Check sheet for the modelled part. Datum: model origin and axes. Units: mm. A direction names the side the tool comes from. Give positions to 0.01 mm unless a question says otherwise; leave off trailing zeros. Loops run counter-clockwise (first coordinate to the right, second up) from the corner with the lowest first, then second, coordinate; pieces in that order, holes last. Notation, with made-up numbers: M -3.5,78.25 L 41.5,78.25 A14 ccw 41.5,89.25 Z; hole C 35.5,-1.5 d8. An arc over 180 degrees is marked long. Use one line per item in the form item = value.
Autodesk Inventor part; units mm, degrees
ref_plane "YZ Plane" through (0, 0, 0) normal (1, 0, 0) x (0, 1, 0)
ref_plane "XZ Plane" through (0, 0, 0) normal (0, 1, 0) x (-1, 0, 0)
ref_plane "XY Plane" through (0, 0, 0) normal (0, 0, 1) x (1, 0, 0)
sketch "スケッチ1" plane through (0, 0, 0) normal (0, 0, 1) x (1, 0, 0)
  line L0 (-16.25, -16.25) -> (16.25, -16.25) construction
  line L1 (16.25, -16.25) -> (16.25, 16.25) construction
  line L2 (16.25, 16.25) -> (-16.25, 16.25) construction
  line L3 (-16.25, 16.25) -> (-16.25, -16.25) construction
  line L4 (-16.25, -16.25) -> (16.25, 16.25) construction
  line L5 (16.25, -16.25) -> (-16.25, 16.25) construction
  line L6 (-8.35, 16.25) -> (-16.25, 16.25)
  line L7 (-16.25, 16.25) -> (-16.25, 8.35)
  line L8 (8.35, 16.25) -> (16.25, 16.25)
  line L9 (16.25, 16.25) -> (16.25, 8.35)
  line L10 (-16.25, -8.35) -> (-16.25, -16.25)
  line L11 (-16.25, -16.25) -> (-8.35, -16.25)
  line L12 (8.35, -16.25) -> (16.25, -16.25)
  line L13 (16.25, -16.25) -> (16.25, -8.35)
  line L14 (-6.25, 16.25) -> (-6.25, 18.25)
  line L15 (-6.25, 18.25) -> (6.25, 18.25)
  line L16 (6.25, 18.25) -> (6.25, 16.25)
  arc A0 (-8.35, 16.25) -> (-6.25, 16.25) centre (-7.3, 16.25) ccw
  arc A1 (6.25, 16.25) -> (8.35, 16.25) centre (7.3, 16.25) ccw
  line L17 (0, 16.25) -> (0, 0) construction
  line L18 (0, 0) -> (16.25, 0) construction
  line L19 (-16.25, 6.25) -> (-18.25, 6.25)
  line L20 (-18.25, 6.25) -> (-18.25, -6.25)
  line L21 (-18.25, -6.25) -> (-16.25, -6.25)
  arc A2 (-16.25, 6.25) -> (-16.25, 8.35) centre (-16.25, 7.3) ccw
  arc A3 (-16.25, -8.35) -> (-16.25, -6.25) centre (-16.25, -7.3) ccw
  line L22 (-6.25, -16.25) -> (-6.25, -18.25)
  line L23 (-6.25, -18.25) -> (6.25, -18.25)
  line L24 (6.25, -18.25) -> (6.25, -16.25)
  arc A4 (-6.25, -16.25) -> (-8.35, -16.25) centre (-7.3, -16.25) ccw
  arc A5 (8.35, -16.25) -> (6.25, -16.25) centre (7.3, -16.25) ccw
  line L25 (16.25, 6.25) -> (18.25, 6.25)
  line L26 (18.25, 6.25) -> (18.25, -6.25)
  line L27 (18.25, -6.25) -> (16.25, -6.25)
  arc A6 (16.25, 8.35) -> (16.25, 6.25) centre (16.25, 7.3) ccw
  arc A7 (16.25, -6.25) -> (16.25, -8.35) centre (16.25, -7.3) ccw
  line L28 (-12.8, 16.25) -> (-9.7, 16.25) construction
  line L29 (-9.7, 16.25) -> (-9.7, 13.25) construction
  line L30 (-9.7, 13.25) -> (-12.8, 13.25) construction
  line L31 (-12.8, 13.25) -> (-12.8, 16.25) construction
  line L32 (-16.25, 12.8) -> (-13.25, 12.8) construction
  line L33 (-13.25, 12.8) -> (-13.25, 9.7) construction
  line L34 (-13.25, 9.7) -> (-16.25, 9.7) construction
  line L35 (-16.25, 9.7) -> (-16.25, 12.8) construction
  line L36 (-10.1287, 12.25) -> (10.1287, 12.25)
  line L37 (10.1287, 12.25) -> (0, 2.1213)
  line L38 (0, 2.1213) -> (-10.1287, 12.25)
  line L39 (-12.25, 10.1287) -> (-12.25, -10.1287)
  line L40 (-12.25, -10.1287) -> (-2.1213, 0)
  line L41 (-2.1213, 0) -> (-12.25, 10.1287)
  line L42 (-10.1287, -12.25) -> (10.1287, -12.25)
  line L43 (10.1287, -12.25) -> (0, -2.1213)
  line L44 (0, -2.1213) -> (-10.1287, -12.25)
  line L45 (12.25, 10.1287) -> (12.25, -10.1287)
  line L46 (12.25, -10.1287) -> (2.1213, 0)
  line L47 (2.1213, 0) -> (12.25, 10.1287)
  line L48 (-11.25, 16.25) -> (-11.25, 13.25) construction
  line L49 (-13.25, 11.25) -> (-16.25, 11.25) construction
  dimension "d0" = 32.5
  dimension "d1" = 1.05
  dimension "d2" = 2
  dimension "d3" = 10
  dimension "d4" = 3.1
  dimension "d6" = 3
  dimension "d8" = 3
  dimension "d9" = 3
  dimension "d10" = 3
  dimension "d11" = 3
  dimension "d12" = 3
  dimension "d13" = 4
  dimension "d17" = 5
  dimension "d18" = 5
extrude "押し出し1" add sketch "スケッチ1" along normal blind 2.5 contours A0 L14 L15 L16 A1 L8 L9 A6 L25 L26 L27 A7 L13 L12 A5 L24 L23 L22 A4 L11 L10 A3 L21 L20 L19 A2 L7 L6 | L36 L37 L38 | L41 L40 L39 | L44 L43 L42 | L45 L46 L47
mirror "ミラー1" about plane through (0, 0, 0) normal (0, 0, -1) of "押し出し1"
fillet "フィレット1" [suppressed]
equation "\"d8\" = d6"
equation "\"d10\" = d9"
equation "\"d11\" = d10"
equation "\"d12\" = d11"
equation "\"d18\" = d17"
properties part number "上腕_メインフレーム_1_1" material "アセタール樹脂、黒"
1) Section check C-C (y = -11.5). Record the cut outline in (x, z), then the cut area to 4 significant figures.
Evaluation:
outline = M -16.25,-2.5 L 16.25,-2.5 L 16.25,2.5 L -16.25,2.5 Z
area = 162.5 mm^2
2) Set-up check for faces 1 (the face through (6.25, -17, 0)), 2 (the face through (-17, 6.25, 0)), 3 (the face through (-16.25, -12, 0)): record each of +Z, -Z, +X, -X, +Y, -Y from which the full face is reachable in a straight line by a thin tool's end or side.
Evaluation:
face_1 = +Z, -Z, +X, -Y
face_2 = +Z, -Z, -X, +Y
face_3 = +Z, -Z, -X, -Y
3) Section check A-A (z = 1.35). Record the cut outline in (x, y).
Evaluation:
outline = M -18.25,-6.25 L -16.25,-6.25 A1.05 cw -16.25,-8.35 L -16.25,-16.25 L -8.35,-16.25 A1.05 cw -6.25,-16.25 L -6.25,-18.25 L 6.25,-18.25 L 6.25,-16.25 A1.05 cw 8.35,-16.25 L 16.25,-16.25 L 16.25,-8.35 A1.05 cw 16.25,-6.25 L 18.25,-6.25 L 18.25,6.25 L 16.25,6.25 A1.05 cw 16.25,8.35 L 16.25,16.25 L 8.35,16.25 A1.05 cw 6.25,16.25 L 6.25,18.25 L -6.25,18.25 L -6.25,16.25 A1.05 cw -8.35,16.25 L -16.25,16.25 L -16.25,8.35 A1.05 cw -16.25,6.25 L -18.25,6.25 Z
4) Release check for a two-part mould opening along X. For faces 4 (the face through (-12, 16.25, 0)), 5 (the face through (-7.3, -15.2, 0)), 6 (the face through (16.25, -12, 0)) record: pulls with the +X half, pulls with the -X half, needs draft (parallel to the pull), parting line crosses it, or undercut.
Evaluation:
face_4 = needs draft
face_5 = undercut
face_6 = pulls with the +X half
5) Scan lines: line 1 (Y direction, x = -14, z = 0.35); line 2 (Y direction, x = 17, z = 1.85). Record each from-to range of solid material in increasing order.
Evaluation:
line_1 = -16.25 to 16.25
line_2 = -6.25 to 6.25
6) Depth check by flat-ended pin: pin 1 Ø0.6 at (y, z) = (17, 0.5) entering from -X; pin 2 Ø0.6 at (x, z) = (-17.5, 0.5) entering from -Y; pin 3 Ø1.5 at (x, z) = (14, 1) entering from -Y. Enter the tip coordinate at first touch or a pass-through.
Evaluation:
pin_1 = -6.25
pin_2 = -6.25
pin_3 = -16.25
7) Section check B-B (x = 7.3). Record the cut outline in (y, z), then the cut area to 3 significant figures.
Evaluation:
outline = M -15.2,-2.5 L 15.2,-2.5 L 15.2,2.5 L -15.2,2.5 Z
area = 152 mm^2
